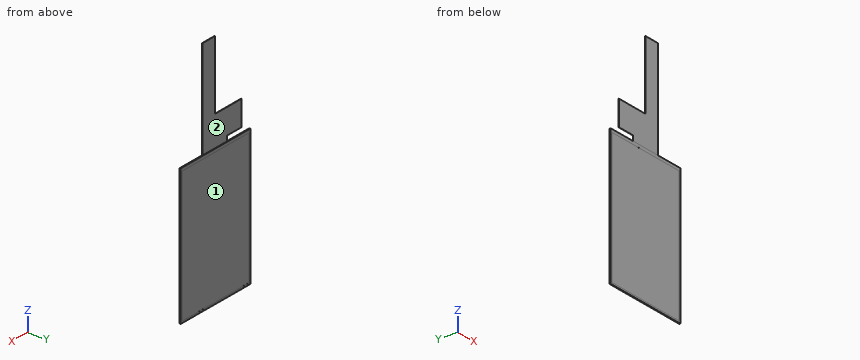
from build123d import *

# Parameters (mm, degrees)
SKETCH1_W           = 84.6
SKETCH1_H           = 135.85
BOSS_EXTRUDE1_DEPTH = 0.946
BOSS_EXTRUDE2_START = 0.01
BOSS_EXTRUDE2_DEPTH = 0.3
SKETCH3_W           = 81
SKETCH3_H           = 131.05
CUT_EXTRUDE1_DEPTH  = 0.01
CUT_EXTRUDE3_START  = -0.946
SKETCH3_2_W         = 81
SKETCH3_2_H         = 131.05
CUT_EXTRUDE3_DEPTH  = 0.01


with BuildPart() as part:
    # Sketch1 → Boss-Extrude1 (new body)
    with BuildSketch(Plane(origin=(0, 0, 0), x_dir=(1, 0, 0), z_dir=(0, 1, 0))):
        with Locations((0, 67.925)):
            Rectangle(SKETCH1_W, SKETCH1_H)
    extrude(amount=BOSS_EXTRUDE1_DEPTH)

    # Sketch2 → Boss-Extrude2 (add)
    with BuildSketch(Plane(origin=(0, 0, 0), x_dir=(1, 0, 0), z_dir=(0, 1, 0)).offset(BOSS_EXTRUDE2_START)):
        Polygon((-15, 0), (-15, -5), (-32.3, -5), (-32.3, -30), (0, -30), (0, -98), (15, -98), (15, 0), align=None)
    extrude(amount=BOSS_EXTRUDE2_DEPTH)

    # Sketch3 → Cut-Extrude1 (cut)
    with BuildSketch(Plane(origin=(0, 0.946, 0), x_dir=(1, 0, 0), z_dir=(0, 1, 0))):
        with Locations((0, 68.525)):
            Rectangle(SKETCH3_W, SKETCH3_H)
    extrude(amount=-CUT_EXTRUDE1_DEPTH, mode=Mode.SUBTRACT)

    # Sketch3<2> → Cut-Extrude3 (cut)
    with BuildSketch(Plane(origin=(0, 0.946, 0), x_dir=(1, 0, 0), z_dir=(0, 1, 0)).offset(CUT_EXTRUDE3_START)):
        with Locations((0, 68.525)):
            Rectangle(SKETCH3_2_W, SKETCH3_2_H)
    extrude(amount=CUT_EXTRUDE3_DEPTH, mode=Mode.SUBTRACT)


solid = part.part
The model under review builds one solid part; all positions refer to its coordinate system, in mm. Face numbers are marked on the shaded views. A direction names the side the tool comes from. Round coordinates to 2 decimals unless told otherwise and drop trailing zeros. Write each loop counter-clockwise with the first axis right and the second up, starting at its lowest first coordinate (ties: lowest second). Pieces come first, ordered by that corner, then holes. Notation, with made-up numbers: (53, 75) -> (105, 75) arc R35 cw to (105, 111) -> close; hole circle Ø8 at (8, 70). An arc over 180 degrees is marked (long way). Answer as a JSON object with one key per item and string values.
1. Clearance check with flat-ended pins moving along their axes: pin 1 (24.5 mm diameter, centred on x = 19, z = -44.5, fed in from +Y); pin 2 (23.5 mm diameter, centred on x = -3.5, z = 57, fed in from -Y). State where each tip first meets the part, or that it passes through.
Results found:
{"pin 1": "stops at y = 0.94", "pin 2": "stops at y = 0.01"}
2. We need section D-D on y = 0.6. State the section outline as (x, z) points, and give its area (3 significant figures).
Results found:
{"outline": "(-42.3, -135.85) -> (42.3, -135.85) -> (42.3, 0) -> (-42.3, 0) -> close", "area": "11,500 mm^2"}
3. Machinability: for the marked faces 1 and 2, which of the approach directions +Z, -Z, +X, -X, +Y, -Y give a long, thin tool a straight path to every point of the face, cutting with its end or side? Answer none if there is none.
Results found:
{"face 1": "+Z, -Z, +X, -X, +Y", "face 2": "+Z, +X, -X, +Y"}
4. To check wall thickness, follow line 1 along Y through (x, z) = (-31, -101); line 2 along X through (y, z) = (0.25, 4); line 3 along Z through (x, y) = (-32.5, 0.1). State the ranges of each line that lie inside material, in increasing order.
Results found:
{"line 1": "y = 0.01 to 0.94", "line 2": "x = -15 to 15", "line 3": "z = -135.85 to 0"}
